Geometry: final body of the model. Coordinates: model frame, mm. Face numbers are marked on the shaded views. Give positions to 0.01 mm unless a question says otherwise; leave off trailing zeros. Write each loop counter-clockwise with the first axis right and the second up, starting at its lowest first coordinate (ties: lowest second). Pieces come first, ordered by that corner, then holes. Notation, with made-up numbers: M 30,-16.5 L 79,-16.5 A20 ccw 79,5.5 Z; hole C -19,52 d7. An arc over 180 degrees is marked long. Use a Markdown table: item, result. Add a question column.
(1) Material intervals for L1, parallel to Y at x = 219, z = 111.95; L2, parallel to X at y = -102.5, z = 127; L3, parallel to Z at x = 74, y = -4, sorted ascending.
(2) Cut plane C-C (x = 181). Output: boundary loops of the cut face in (y, z), plus the area to 3 significant figures.
(3) Cut plane A-A (y = -28). Output: boundary loops of the cut face in (x, z), plus the area to 3 significant figures.
(4) Cut plane B-B (z = 139). Output: boundary loops of the cut face in (x, y).
(5) Pin query (flat end, axial travel): pin 1 Ø0.6 at (x, z) = (219, 112.5) entering from -Y; pin 2 Ø2 at (x, z) = (217.5, 111.5) entering from +Y; pin 3 Ø3.5 at (x, y) = (220.5, -121) entering from +Z. Return the tip coordinate at first contact, or that it passes through.
(6) Draft query along X for the marked faces 1, 2 and 3. Return one class per face: released by +X, released by -X, zero draft, split by the parting line, or undercut.
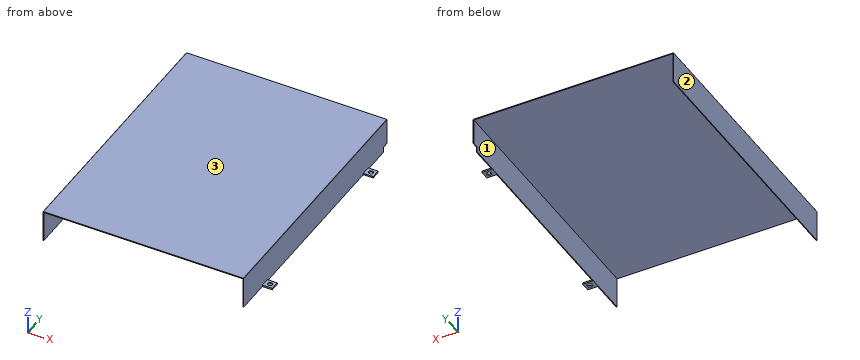
```python
from build123d import *

# Parameters (mm, degrees)
WYCI_GNI_CIE_CIENKA_CIANKA1_DEPTH      = 172
WYCI_GNI_CIE_CIENKA_CIANKA1_DEPTH_BACK = 172
SZKIC2_W                               = 13
SZKIC2_H                               = 12
SZKIC2_R                               = 3
DODANIE_WYCI_GNI_CIE1_DEPTH            = 2
ZAOKR_GLENIE1_R                        = 0.5
WYTNIJ_WYCI_GNI_CIE2_DEPTH             = 14
WYTNIJ_WYCI_GNI_CIE2_DEPTH_BACK        = 2
ZAOKR_GLENIE4_R                        = 0.5
ZAOKR_GLENIE5_R                        = 0.5


with BuildPart() as part:
    # Szkic1 → Wyciągnięcie-cienka ścianka1 (new body, two sides)
    with BuildSketch(Plane(origin=(0, 0, 0), x_dir=(1, 0, 0), z_dir=(0, 1, 0))) as wyci_gni_cie_cienka_cianka1_sk:
        Polygon((211, -111), (211, -152), (-51, -152), (-51, -111), (-52, -111), (-52, -153), (212, -153), (212, -111), align=None)
    extrude(amount=WYCI_GNI_CIE_CIENKA_CIANKA1_DEPTH)
    extrude(wyci_gni_cie_cienka_cianka1_sk.sketch, amount=-WYCI_GNI_CIE_CIENKA_CIANKA1_DEPTH_BACK)

    # Szkic2 → Dodanie-wyciągnięcie1 (add)
    with BuildSketch(Plane(origin=(0, 0, 111), x_dir=(-1, 0, 0), z_dir=(0, 0, -1))):
        with Locations((-218.5, -121)):
            Rectangle(SZKIC2_W, SZKIC2_H)
        with Locations((-219, -121)):
            Circle(SZKIC2_R, mode=Mode.SUBTRACT)
        with Locations((-218.5, 121)):
            Rectangle(SZKIC2_W, SZKIC2_H)
        with Locations((-219, 121)):
            Circle(SZKIC2_R, mode=Mode.SUBTRACT)
    extrude(amount=-DODANIE_WYCI_GNI_CIE1_DEPTH)

    # Zaokrąglenie1
    zaokr_glenie1_edges = [part.edges().sort_by_distance(p)[0] for p in [
        (212, 0, 153),
        (-52, 0, 153),
    ]]
    fillet(zaokr_glenie1_edges, radius=ZAOKR_GLENIE1_R)

    # Szkic5 → Wytnij-wyciągnięcie2 (cut, two sides)
    with BuildSketch(Plane(origin=(212, 0, 0), x_dir=(0, 0, -1), z_dir=(1, 0, 0))) as wytnij_wyci_gni_cie2_sk:
        Polygon((-118, 873.551878025), (-118, 172), (-118, 164), (-111, 164), (590.551878025, 164), (1583.395439141, 1155.444306753), (874.843561116, 1864.996184778), align=None)
    extrude(amount=WYTNIJ_WYCI_GNI_CIE2_DEPTH, mode=Mode.SUBTRACT)
    extrude(wytnij_wyci_gni_cie2_sk.sketch, amount=-WYTNIJ_WYCI_GNI_CIE2_DEPTH_BACK, mode=Mode.SUBTRACT)

    # Zaokrąglenie4
    zaokr_glenie4_edges = [part.edges().sort_by_distance(p)[0] for p in [
        (211.5, 164, 118),
    ]]
    fillet(zaokr_glenie4_edges, radius=ZAOKR_GLENIE4_R)

    # Zaokrąglenie5
    zaokr_glenie5_edges = [part.edges().sort_by_distance(p)[0] for p in [
        (212, 164, 114.25),
        (212, 168.25, 118),
        (212, 164.146446609, 117.853553391),
    ]]
    fillet(zaokr_glenie5_edges, radius=ZAOKR_GLENIE5_R)


solid = part.part
```
Answer list:
| question | item | result |
|---|---|---|
| 1 | L1 | -127 to -124, -118 to -115, 115 to 118, 124 to 127 |
| 1 | L2 | -52 to -51, 211 to 212 |
| 1 | L3 | 152 to 153 |
| 2 | outline | M -172,152 L 172,152 L 172,153 L -172,153 Z |
| 2 | area | 344 mm² |
| 3 | outline | M -52,111 L -51,111 L -51,152 L 211,152 L 211,111 L 212,111 L 212,152.5 A0.5 ccw 211.5,153 L -51.5,153 A0.5 ccw -52,152.5 Z |
| 3 | area | 346 mm² |
| 4 | outline | M -52,-172 L -51,-172 L -51,172 L -52,172 Z; M 211,-172 L 212,-172 L 212,172 L 211,172 Z |
| 5 | pin 1 | y = -127 |
| 5 | pin 2 | y = 127 |
| 5 | pin 3 | z = 113 |
| 6 | face 1 | undercut |
| 6 | face 2 | released by -X |
| 6 | face 3 | zero draft |
